Could you check a few things on this model? Use its own coordinates, in mm. A direction names the side the tool comes from. Give positions to 0.01 mm unless a question says otherwise; leave off trailing zeros. Write each loop counter-clockwise with the first axis right and the second up, starting at its lowest first coordinate (ties: lowest second). Pieces come first, ordered by that corner, then holes. Notation, with made-up numbers: (78.5, 53.25) - (103.5, 53.25) arc R27 cw to (103.5, 72.25) - close; hole circle Ø7 at (-13.75, 78). An arc over 180 degrees is marked (long way). Answer in a Markdown table with one row per item.
from build123d import *

# Parameters (mm, degrees)
F0_R      = 1.5
F0_R_2    = 1
F0_R_3    = 1.2
F1_DEPTH  = 11.5
F2_R      = 3
F2_R_2    = 2.4
F3_DEPTH  = 25
F4_DEPTH  = 25
F5_DEPTH  = 3.5
F6_DEPTH  = 2
F7_SIZE   = 0.5
F10_ANGLE = 180


with BuildPart() as f1:
    # F0 (on Front) → F1 (new body)
    with BuildSketch(Plane.XZ):
        with BuildLine():
            Line((-6.8, -20), (4.5, -20))
            Line((4.5, -20), (4.5, 0))
            Line((4.5, 0), (-15.5, 0))
            Line((-15.5, 0), (-15.5, -18.5))
            Line((-15.5, -18.5), (-8.3, -18.5))
            ThreePointArc((-8.3, -18.5), (-7.7343145751, -18.7343145751), (-7.5, -19.3))
            ThreePointArc((-7.5, -19.3), (-7.2949747468, -19.7949747468), (-6.8, -20))
        make_face()
        with Locations((-13, -14.5)):
            Circle(F0_R, mode=Mode.SUBTRACT)
        with Locations((-13, -5.5)):
            Circle(F0_R, mode=Mode.SUBTRACT)
        with Locations((-4, -8)):
            Circle(F0_R, mode=Mode.SUBTRACT)
        with Locations((-4, -4.5)):
            Circle(F0_R_2, mode=Mode.SUBTRACT)
        with Locations((-4, -8)):
            Circle(F0_R)
        with Locations((-4, -8)):
            Circle(F0_R_3, mode=Mode.SUBTRACT)
        with Locations((-13, -5.5)):
            Circle(F0_R)
        with Locations((-13, -5.5)):
            Circle(F0_R_3, mode=Mode.SUBTRACT)
        with Locations((-13, -14.5)):
            Circle(F0_R)
        with Locations((-13, -14.5)):
            Circle(F0_R_3, mode=Mode.SUBTRACT)
        with Locations((-4, -8)):
            Circle(F0_R_3)
        with Locations((-13, -5.5)):
            Circle(F0_R_3)
        with Locations((-13, -14.5)):
            Circle(F0_R_3)
        with Locations((-4, -4.5)):
            Circle(F0_R_2)
    extrude(amount=F1_DEPTH)

    # F2 (on Top) → F3 (cut)
    with BuildSketch(Plane.XY):
        with BuildLine():
            Line((-10.4432125306, -6.7), (-15.5, -6.7))
            Line((-15.5, -6.7), (-15.5, -8.3))
            Line((-15.5, -8.3), (-10.4432125306, -8.3))
            ThreePointArc((-10.4432125306, -8.3), (-4.45, -7.5), (-10.4432125306, -6.7))
        make_face()
        with Locations((0, -7)):
            Circle(F2_R)
        with Locations((0, -7)):
            Circle(F2_R_2, mode=Mode.SUBTRACT)
        with Locations((0, -7)):
            Circle(F2_R_2)
    extrude(amount=-F3_DEPTH, mode=Mode.SUBTRACT)

    # F0 (on Front) → F4 (cut)
    with BuildSketch(Plane.XZ):
        with Locations((-13, -5.5)):
            Circle(F0_R)
        with Locations((-13, -5.5)):
            Circle(F0_R_3, mode=Mode.SUBTRACT)
        with Locations((-13, -14.5)):
            Circle(F0_R)
        with Locations((-13, -14.5)):
            Circle(F0_R_3, mode=Mode.SUBTRACT)
        with Locations((-13, -5.5)):
            Circle(F0_R_3)
        with Locations((-13, -14.5)):
            Circle(F0_R_3)
    extrude(amount=F4_DEPTH, mode=Mode.SUBTRACT)

    # F0 (on Front) → F5 (cut)
    with BuildSketch(Plane.XZ):
        with Locations((-4, -8)):
            Circle(F0_R)
        with Locations((-4, -8)):
            Circle(F0_R_3, mode=Mode.SUBTRACT)
        with Locations((-4, -8)):
            Circle(F0_R_3)
    extrude(amount=F5_DEPTH, mode=Mode.SUBTRACT)

    # F0 (on Front) → F6 (cut)
    with BuildSketch(Plane.XZ):
        with Locations((-4, -4.5)):
            Circle(F0_R_2)
    extrude(amount=F6_DEPTH, mode=Mode.SUBTRACT)

    # F7
    f7_edges = [f1.edges().sort_by_distance(p)[0] for p in [
        (4.5, -5.75, 0),
        (-5.5, -11.5, 0),
        (-15.5, -9.9, 0),
        (-15.5, -3.35, 0),
        (-5.5, 0, 0),
        (4.5, -11.5, -10),
        (-15.5, -11.5, -9.25),
        (-11.9, -11.5, -18.5),
        (-7.734315, -11.5, -18.734315),
        (-7.294975, -11.5, -19.794975),
        (-1.15, -11.5, -20),
        (4.5, -5.75, -20),
        (-15.5, -9.9, -18.5),
        (-15.5, -3.35, -18.5),
        (4.5, 0, -10),
        (-1.15, 0, -20),
        (-7.294975, 0, -19.794975),
        (-7.734315, 0, -18.734315),
        (-11.9, 0, -18.5),
        (-15.5, 0, -9.25),
    ]]
    chamfer(f7_edges, length=F7_SIZE)


with BuildPart() as f8_1:
    # F8: instance of F1
    add(f1.part.mirror(Plane.XZ))


with BuildPart() as f8_1_1:
    # F10: moved
    add(f8_1.part.rotate(Axis((-5.5, 0, -0.5), (1, 0, 0)), F10_ANGLE))


solid = f8_1_1.part
1) Imagine slicing it at B-B (x = -13). List the corners of the cut face in (y, z) for me.
Check values:
| item | result |
|---|---|
| outline | (-11.5, -0.5) - (-11, -1) - (-8.3, -1) - (-8.3, 3) - (-11.5, 3) - close; (-11.5, 6) - (-8.3, 6) - (-8.3, 12) - (-11.5, 12) - close; (-11.5, 15) - (-8.3, 15) - (-8.3, 17.5) - (-11, 17.5) - (-11.5, 17) - close; (-6.7, -1) - (-0.5, -1) - (0, -0.5) - (0, 3) - (-6.7, 3) - close; (-6.7, 6) - (0, 6) - (0, 12) - (-6.7, 12) - close; (-6.7, 15) - (0, 15) - (0, 17) - (-0.5, 17.5) - (-6.7, 17.5) - close |
2) Imagine slicing it at C-C (z = 7). List the corners of the cut face in (x, y) for me, then the cut area to 3 significant figures.
Check values:
| item | result |
|---|---|
| outline | (-15.5, -11) - (-15, -11.5) - (4, -11.5) - (4.5, -11) - (4.5, -0.5) - (4, 0) - (-2.5, 0) - (-2.5, -3.5) - (-5.5, -3.5) - (-5.5, 0) - (-15, 0) - (-15.5, -0.5) - (-15.5, -6.7) - (-10.44, -6.7) arc R3.05 cw (long way) to (-10.44, -8.3) - (-15.5, -8.3) - close; hole circle Ø6 at (0, -7) |
| area | 154 mm2 |
3) Imagine slicing it at A-A (z = 13.5). List the corners of the cut face in (x, y) for me.
Check values:
| item | result |
|---|---|
| outline | (-15.5, -11) - (-15, -11.5) - (-14.5, -11.5) - (-14.5, -8.3) - (-15.5, -8.3) - close; (-15.5, -6.7) - (-14.5, -6.7) - (-14.5, 0) - (-15, 0) - (-15.5, -0.5) - close; (-11.5, -11.5) - (4, -11.5) - (4.5, -11) - (4.5, -0.5) - (4, 0) - (-11.5, 0) - (-11.5, -6.7) - (-10.44, -6.7) arc R3.05 cw (long way) to (-10.44, -8.3) - (-11.5, -8.3) - close; hole circle Ø6 at (0, -7) |
4) Will these pins go through, and if not, where does the flat tip stop? P1, Ø4, axis at x = -13, z = 13.5, coming from the -Y side; P2, Ø1, axis at x = -2, y = -8, coming from the -Z side; P3, Ø0.9, axis at x = -4, z = 7, coming from the +Y side; P4, Ø2, axis at x = -11.5, y = -9, coming from the +Z side.
Check values:
| item | result |
|---|---|
| P1 | stops at y = -11.5 |
| P2 | passes through |
| P3 | stops at y = -3.5 |
| P4 | stops at z = 17.5 |
5) We'd pull the mould along Y, two halves only. Please class faces 1 (the face through (-5, -5, -1)), 2 (the face through (-6, -11.5, 9)), 3 (the face through (-4.452, -7.623, 8.86)): +Y half, -Y half, draft (parallel to the pull), parting line (faces both ways), or undercut.
Check values:
| item | result |
|---|---|
| face 1 | draft |
| face 2 | -Y half |
| face 3 | undercut |
6) If I drill on line 1 (Z direction, x = -13, y = -9.7); line 2 (Y direction, x = -7.5, z = 5.5); line 3 (X direction, y = -9, z = 12.5), over which ranges is the centre line in solid material (lowest first)?
Check values:
| item | result |
|---|---|
| line 1 | z = -1 to 3, 6 to 12, 15 to 17.5 |
| line 2 | y = -11.5 to -10.55, -4.45 to 0 |
| line 3 | x = -15.5 to -14.12, -11.88 to -10.16, -4.84 to -2.24, 2.24 to 4.5 |
7) On a 3-axis mill with a long thin cutter (end or side, diameter ignored), from which of +Z, -Z, +X, -X, +Y, -Y can I reach the whole of each face in a straight line? I mean faces 4 (the face through (-4, -3.5, 7)), 5 (the face through (-15.5, -10, 8)), 6 (the face through (-13, -6.7, 8)). Say none if no direction works.
Check values:
| item | result |
|---|---|
| face 4 | +Y |
| face 5 | +Z, -Z, -X, +Y, -Y |
| face 6 | +Z, -Z, -X |
8) Imagine slicing it at D-D (x = 0). List the corners of the cut face in (y, z) for me, then the cut area to 4 significant figures.
Check values:
| item | result |
|---|---|
| outline | (-11.5, -0.5) - (-11, -1) - (-10, -1) - (-10, 19) - (-11, 19) - (-11.5, 18.5) - close; (-4, -1) - (-0.5, -1) - (0, -0.5) - (0, 18.5) - (-0.5, 19) - (-4, 19) - close |
| area | 109.5 mm2 |
